The model under review builds one solid part; all positions refer to its coordinate system, in mm. A direction names the side the tool comes from. Coordinates: 2 decimals unless noted, no trailing zeros. Loops run counter-clockwise (first coordinate to the right, second up) from the corner with the lowest first, then second, coordinate; pieces in that order, holes last. Notation, with made-up numbers: (-36.5, 1.5) - (-4.5, 1.5) arc R14 ccw to (-4.5, 17.5) - close; hole circle Ø5 at (41.25, 71.25). An arc over 180 degrees is marked (long way). Use a Markdown table: item, result. Add a question column.
1) Add section C-C, the plane z = 44.5. Give the boundary of the cut face in (x, y) (3 decimals).
2) Add section D-D, the plane x = 25.4. Give the boundary of the cut face in (y, z), and give its area (3 significant figures).
3) For faces 1 (the cylindrical face through (42.43, 7.44, 9.55)), 2 (the cylindrical face through (10.957, 41.387, 86.985)), 3 (the flat face through (25, 0, 49)), 4 (the flat face through (18, 18, 43.18)), 5 (the cylindrical face through (8.37, 5.83, 90.18)), list the 3-axis set-ups (+Z, -Z, +X, -X, +Y, -Y) from which the entire face can be reached by the end or side of a thin tool; tool diameter is ignored.
4) The part is to be moulded in two halves that separate along Z. For faces 6 (the flat face through (8, 26, 0)), 7 (the conical face through (33.02, 5.55, 87.22)), 8 (the flat face through (50.8, 25, 49)), say which applies: pulls with the +Z half, pulls with the -Z half, needs draft (parallel to the pull), parting line crosses it, or undercut.
5) Clearance check with flat-ended pins moving along their axes: pin 1 (4 mm diameter, centred on y = 41.275, z = 64.135, fed in from +X); pin 2 (6.5 mm diameter, centred on y = 41.275, z = 89.535, fed in from +X) (3 decimals); pin 3 (5.5 mm diameter, centred on y = 39, z = 89.5, fed in from +X); pin 4 (5.5 mm diameter, centred on y = 46.355, z = 25, fed in from +X). State where each tip first meets the part, or that it passes through.
6) Add section B-B, the plane y = 25.4. Give the boundary of the cut face in (x, z), and give its area (3 significant figures).
7) To check wall thickness, follow L1, parallel to Z at x = 33, y = 43; L2, parallel to Y at x = 31.5, z = 73.5; L3, parallel to Y at x = 17, z = 90 (3 decimals). State the ranges of each line that lie inside material, in increasing order. Write a range as [from, to].
8) Add section A-A, the plane z = 25. Give the number of separate pieces and of enclosed holes in the cut face, and give its area (3 significant figures).
```python
from build123d import *

# Parameters (mm, degrees)
SKETCH1_W                                    = 50.8
SKETCH1_H                                    = 50.8
BOSS_EXTRUDE1_DEPTH                          = 99.06
SKETCH2_R                                    = 16.75
CUT_EXTRUDE1_DEPTH                           = 43.18
SKETCH3_R                                    = 9.5504
CUT_EXTRUDE2_DEPTH                           = 92.015682165
SKETCH6_W                                    = 6.35
SKETCH6_H                                    = 25.4
CUT_EXTRUDE3_DEPTH                           = 123.36896502
CBORE_START                                  = 28.575
CBORE_FOR_1_4_SOCKET_HEAD_CAP_SCREW1_OUT_R   = 3.3782
CBORE_FOR_1_4_SOCKET_HEAD_CAP_SCREW1_DEPTH   = 22.225
CBORE_START_2                                = 44.45
CBORE_FOR_1_4_SOCKET_HEAD_CAP_SCREW1_2_O_R   = 5.55625
CBORE_FOR_1_4_SOCKET_HEAD_CAP_SCREW1_2_O_R_2 = 3.3782
CBORE_FOR_1_4_SOCKET_HEAD_CAP_SCREW1_2_DEPTH = 6.35
F_1_4_20_TAPPED_HOLE1_D                      = 5.1054
CBORE_FOR_6_SOCKET_HEAD_CAP_SCREW1_OUTL_R    = 1.89865
CBORE_FOR_6_SOCKET_HEAD_CAP_SCREW1_DEPTH     = 22.225
CBORE_START_3                                = 47.2948
CBORE_FOR_6_SOCKET_HEAD_CAP_SCREW1_2_OU_R    = 3.57251
CBORE_FOR_6_SOCKET_HEAD_CAP_SCREW1_2_OU_R_2  = 1.89865
CBORE_FOR_6_SOCKET_HEAD_CAP_SCREW1_2_DEPTH   = 3.5052
F_6_32_TAPPED_HOLE1_D                        = 2.7051
F_1_4_20_TAPPED_HOLE2_D                      = 5.1054
F_1_4_20_TAPPED_HOLE2_DEPTH                  = 16.51
F_1_4_20_TAPPED_HOLE2_TIP                    = 1.533816902
F_1_4_20_TAPPED_HOLE3_D                      = 5.1054
F_1_4_20_TAPPED_HOLE3_DEPTH                  = 16.51
F_1_4_20_TAPPED_HOLE3_TIP                    = 1.533816902


# Read off the part's stored shape, not the designer's step: CBORE for 1/4 Socket Head Cap Screw1, CBORE for #6 Socket Head Cap Screw1
with BuildPart() as part:
    # Sketch1 → Boss-Extrude1 (new body)
    with BuildSketch(Plane.XY):
        with Locations((25.4, 25.4)):
            Rectangle(SKETCH1_W, SKETCH1_H)
    extrude(amount=BOSS_EXTRUDE1_DEPTH)

    # Sketch2 → Cut-Extrude1 (cut)
    with BuildSketch(Plane(origin=(0, 0, 0), x_dir=(-1, 0, 0), z_dir=(0, 0, -1))):
        with Locations((-25.4, 25.4)):
            Circle(SKETCH2_R)
    extrude(amount=-CUT_EXTRUDE1_DEPTH, mode=Mode.SUBTRACT)

    # Sketch3 → Cut-Extrude2 (cut, through all)
    with BuildSketch(Plane(origin=(0, 0, 43.18), x_dir=(-1, 0, 0), z_dir=(0, 0, -1))):
        with Locations((-25.4, 25.4)):
            Circle(SKETCH3_R)
    extrude(amount=-CUT_EXTRUDE2_DEPTH, mode=Mode.SUBTRACT)

    # Sketch6 → Cut-Extrude3 (cut, through all)
    with BuildSketch(Plane(origin=(0, 0, 0), x_dir=(-1, 0, 0), z_dir=(0, 0, -1))):
        with Locations((-25.4, 38.1)):
            Rectangle(SKETCH6_W, SKETCH6_H)
    extrude(amount=-CUT_EXTRUDE3_DEPTH, mode=Mode.SUBTRACT)

    # CBORE for 1/4 Socket Head Cap Screw1 out → CBORE for 1/4 Socket Head Cap Screw1 (cut)
    with BuildSketch(Plane.YZ.offset(CBORE_START)):
        with Locations((41.275, 64.135)):
            Circle(CBORE_FOR_1_4_SOCKET_HEAD_CAP_SCREW1_OUT_R)
        with Locations((41.275, 89.535)):
            Circle(CBORE_FOR_1_4_SOCKET_HEAD_CAP_SCREW1_OUT_R)
    extrude(amount=CBORE_FOR_1_4_SOCKET_HEAD_CAP_SCREW1_DEPTH, mode=Mode.SUBTRACT)

    # CBORE for 1_4 Socket Head Cap Screw1 2 o → CBORE for 1_4 Socket Head Cap Screw1 2 (cut)
    # profile 1 of 2: a face of its own
    with BuildSketch(Plane.YZ.offset(CBORE_START_2)):
        with Locations((41.275, 64.135)):
            Circle(CBORE_FOR_1_4_SOCKET_HEAD_CAP_SCREW1_2_O_R)
        with Locations((41.275, 64.135)):
            Circle(CBORE_FOR_1_4_SOCKET_HEAD_CAP_SCREW1_2_O_R_2, mode=Mode.SUBTRACT)
    # profile 2 of 2: a face of its own
    with BuildSketch(Plane.YZ.offset(CBORE_START_2)):
        with Locations((41.275, 89.535)):
            Circle(CBORE_FOR_1_4_SOCKET_HEAD_CAP_SCREW1_2_O_R)
        with Locations((41.275, 89.535)):
            Circle(CBORE_FOR_1_4_SOCKET_HEAD_CAP_SCREW1_2_O_R_2, mode=Mode.SUBTRACT)
    extrude(amount=CBORE_FOR_1_4_SOCKET_HEAD_CAP_SCREW1_2_DEPTH, mode=Mode.SUBTRACT)

    # 1/4-20 Tapped Hole1 (through all)
    with Locations(Plane(origin=(22.225, 0, 0), x_dir=(0, 0, -1), z_dir=(1, 0, 0))):
        with Locations((-89.535, 41.275), (-64.135, 41.275)):
            Hole(F_1_4_20_TAPPED_HOLE1_D / 2)

    # CBORE for #6 Socket Head Cap Screw1 outl → CBORE for #6 Socket Head Cap Screw1 (cut)
    with BuildSketch(Plane.YZ.offset(CBORE_START)):
        with Locations((46.355, 25)):
            Circle(CBORE_FOR_6_SOCKET_HEAD_CAP_SCREW1_OUTL_R)
    extrude(amount=CBORE_FOR_6_SOCKET_HEAD_CAP_SCREW1_DEPTH, mode=Mode.SUBTRACT)

    # CBORE for _6 Socket Head Cap Screw1 2 ou → CBORE for _6 Socket Head Cap Screw1 2 (cut)
    with BuildSketch(Plane.YZ.offset(CBORE_START_3)):
        with Locations((46.355, 25)):
            Circle(CBORE_FOR_6_SOCKET_HEAD_CAP_SCREW1_2_OU_R)
        with Locations((46.355, 25)):
            Circle(CBORE_FOR_6_SOCKET_HEAD_CAP_SCREW1_2_OU_R_2, mode=Mode.SUBTRACT)
    extrude(amount=CBORE_FOR_6_SOCKET_HEAD_CAP_SCREW1_2_DEPTH, mode=Mode.SUBTRACT)

    # #6-32 Tapped Hole1 (through all)
    with Locations(Plane(origin=(22.225, 0, 0), x_dir=(0, 0, -1), z_dir=(1, 0, 0))):
        with Locations((-25, 46.355)):
            Hole(F_6_32_TAPPED_HOLE1_D / 2)

    # 1/4-20 Tapped Hole2
    with Locations(Plane(origin=(50.8, 0, 0), x_dir=(0, 0, -1), z_dir=(1, 0, 0))):
        with Locations((-87.63, 5.715), (-49.53, 5.715), (-11.43, 5.715)):
            Hole(F_1_4_20_TAPPED_HOLE2_D / 2, depth=F_1_4_20_TAPPED_HOLE2_DEPTH)
            with Locations((0, 0, -(F_1_4_20_TAPPED_HOLE2_DEPTH + F_1_4_20_TAPPED_HOLE2_TIP / 2))):  # 118° drill point
                Cone(0, F_1_4_20_TAPPED_HOLE2_D / 2, F_1_4_20_TAPPED_HOLE2_TIP, mode=Mode.SUBTRACT)

    # 1/4-20 Tapped Hole3
    with Locations(Plane.ZY):
        with Locations((11.43, 5.715), (49.53, 5.715), (87.63, 5.715)):
            Hole(F_1_4_20_TAPPED_HOLE3_D / 2, depth=F_1_4_20_TAPPED_HOLE3_DEPTH)
            with Locations((0, 0, -(F_1_4_20_TAPPED_HOLE3_DEPTH + F_1_4_20_TAPPED_HOLE3_TIP / 2))):  # 118° drill point
                Cone(0, F_1_4_20_TAPPED_HOLE3_D / 2, F_1_4_20_TAPPED_HOLE3_TIP, mode=Mode.SUBTRACT)


solid = part.part
```
From the geometry:
| question | item | result |
|---|---|---|
| 1 | outline | (0, 0) - (50.8, 0) - (50.8, 50.8) - (28.575, 50.8) - (28.575, 34.407) arc R9.55 cw (long way) to (22.225, 34.407) - (22.225, 50.8) - (0, 50.8) - close |
| 2 | outline | (0, 0) - (8.65, 0) - (8.65, 43.18) - (15.85, 43.18) - (15.85, 99.06) - (0, 99.06) - close |
| 2 | area | 1,260 mm^2 |
| 3 | face 1 | +X |
| 3 | face 2 | +X, -X |
| 3 | face 3 | +Z, -Z, +X, -X, -Y |
| 3 | face 4 | -Z |
| 3 | face 5 | -X |
| 4 | face 6 | pulls with the -Z half |
| 4 | face 7 | undercut |
| 4 | face 8 | needs draft |
| 5 | pin 1 | passes through |
| 5 | pin 2 | stops at x = 22.225 |
| 5 | pin 3 | stops at x = 44.45 |
| 5 | pin 4 | stops at x = 47.29 |
| 6 | outline | (0, 0) - (8.65, 0) - (8.65, 43.18) - (15.85, 43.18) - (15.85, 99.06) - (0, 99.06) - close; (34.95, 43.18) - (42.15, 43.18) - (42.15, 0) - (50.8, 0) - (50.8, 99.06) - (34.95, 99.06) - close |
| 6 | area | 2,520 mm^2 |
| 7 | L1 | z = [0, 61.23], [67.04, 86.63], [92.44, 99.06] |
| 7 | L2 | y = [0, 18.05], [32.75, 50.8] |
| 7 | L3 | y = [0, 20.856], [29.944, 38.765], [43.785, 50.8] |
| 8 | separate pieces | 3 |
| 8 | enclosed holes | 0 |
| 8 | area | 1,490 mm^2 |
